The model under review builds one solid part; all positions refer to its coordinate system, in mm. A direction names the side the tool comes from. Give positions to 0.01 mm unless a question says otherwise; leave off trailing zeros. Order: outer loops, then holes, each group sorted by start corner. A loop starts at its lowest first (then second) coordinate and runs counter-clockwise, first axis right, second up. Notation, with made-up numbers: (85.5, -14.75) - (105.5, -14.75) arc R11 cw to (105.5, 2.25) - close; hole circle Ø11 at (66, -30.5). An arc over 180 degrees is marked (long way). Answer as CSV lines item,"result". Start each with the question number.
from build123d import *

# Parameters (mm, degrees)
BOSS_EXTRUDE1_DEPTH     = 8
SKETCH3_OUTSIDE_W       = 33.14
SKETCH3_OUTSIDE_H       = 32.15
SKETCH3_OUTSIDE_R       = 3.2
CUT_EXTRUDE1_DEPTH      = 10
CUT_EXTRUDE1_DRAFT      = -45
MIRROR2_COPY_1_SKETCH_W = 33.14
MIRROR2_COPY_1_SKETCH_H = 32.15
MIRROR2_COPY_1_SKETCH_R = 3.2
MIRROR2_COPY_1_DEPTH    = 10
MIRROR2_COPY_1_DRAFT    = -45


with BuildPart() as part:
    # Sketch1 → Boss-Extrude1 (new, symmetric)
    with BuildSketch(Plane(origin=(0, 0, 0), x_dir=(1, 0, 0), z_dir=(0, 1, 0))):
        Polygon((3.695041723, 0), (1.847520861, 3.2), (-1.847520861, 3.2), (-3.695041723, 0), (-1.847520861, -3.2), (1.847520861, -3.2), align=None)
    extrude(amount=BOSS_EXTRUDE1_DEPTH, both=True)


with BuildPart() as cut_extrude1_tool:
    # Sketch3 outside → Cut-Extrude1 (with draft: the straight prism first)
    with BuildSketch(Plane(origin=(0, 8, 0), x_dir=(1, 0, 0), z_dir=(0, 1, 0))):
        Rectangle(SKETCH3_OUTSIDE_W, SKETCH3_OUTSIDE_H)
        Circle(SKETCH3_OUTSIDE_R, mode=Mode.SUBTRACT)
    extrude(amount=-CUT_EXTRUDE1_DEPTH)
    # Cut-Extrude1: the draft: its side faces are tilted about the plane it starts from
    cut_extrude1_sides = [cut_extrude1_tool.faces().sort_by_distance(p)[0] for p in [
        (0, 3, 16.075),
        (16.57, 3, 0),
        (0, 3, -16.075),
        (-16.57, 3, 0),
        (-3.2, 3, 0),
    ]]
    draft(cut_extrude1_sides, Plane(origin=(0, 8, 0), x_dir=(1, 0, 0), z_dir=(0, 1, 0)), CUT_EXTRUDE1_DRAFT)


with BuildPart() as part_1:
    add(part.part)

    # Cut-Extrude1: cut by cut_extrude1_tool
    add(cut_extrude1_tool.part, mode=Mode.SUBTRACT)


with BuildPart() as mirror2_copy_1_tool:
    # Mirror2 copy 1 sketch → Mirror2 copy 1 (with draft: the straight prism first)
    with BuildSketch(Plane.XZ.offset(8)):
        Rectangle(MIRROR2_COPY_1_SKETCH_W, MIRROR2_COPY_1_SKETCH_H)
        Circle(MIRROR2_COPY_1_SKETCH_R, mode=Mode.SUBTRACT)
    extrude(amount=-MIRROR2_COPY_1_DEPTH)
    # Mirror2 copy 1: the draft: its side faces are tilted about the plane it starts from
    mirror2_copy_1_sides = [mirror2_copy_1_tool.faces().sort_by_distance(p)[0] for p in [
        (0, -3, 16.075),
        (16.57, -3, 0),
        (0, -3, -16.075),
        (-16.57, -3, 0),
        (-3.2, -3, 0),
    ]]
    draft(mirror2_copy_1_sides, Plane.XZ.offset(8), MIRROR2_COPY_1_DRAFT)


with BuildPart() as part_2:
    add(part_1.part)

    # Mirror2 copy 1: cut by mirror2_copy_1_tool
    add(mirror2_copy_1_tool.part, mode=Mode.SUBTRACT)

    # Sketch2 → M2.5 Tapped Hole1 (revolve, cut)
    with BuildSketch(Plane(origin=(0, 8, 0), x_dir=(0, 0, 1), z_dir=(1, 0, 0))):
        Polygon((0, 0), (0, 6.965882135), (1.025, 6.35), (1.025, 0), align=None)
    m2_5_tapped_hole1 = revolve(axis=Axis((0, 14.35, 0), (0, -1, 0)), mode=Mode.SUBTRACT)

    # Mirror1: M2.5 Tapped Hole1 across plane
    add(m2_5_tapped_hole1.mirror(Plane.ZX), mode=Mode.SUBTRACT)


solid = part_2.part
Item 1: Mouldability with a two-part tool opening along Z and no side actions: class faces 1 (the face through (1.65, -7.88, -2.88)), 2 (the face through (-2.784, 0.112, 1.578)), 3 (the face through (-0.05, 1.14, 0.17)), 4 (the face through (-0.05, -1.14, 0.17)) as released by +Z, released by -Z, zero draft, split by the parting line, or undercut.
Item 2: Machinability: for faces 5 (the face through (1.67, -7.88, 2.87)), 6 (the face through (-1.016, 4.869, -0.133)), which of the approach directions +Z, -Z, +X, -X, +Y, -Y give a long, thin tool a straight path to every point of the face, cutting with its end or side? Answer none if there is none.
Item 3: For line 1 along Z through (x, y) = (0, 4) (3 decimals); line 2 along X through (y, z) = (-5.5, 0.5); line 3 along X through (y, z) = (1.5, 0.25), list the stretches that pass through material, from the lowest coordinate up.
Item 4: Take a section at B-B on y = 0.25. Write out the cut boundary in (x, z), and give its area (3 significant figures).
Item 5: Take a section at A-A on y = -6.5. Write out the cut boundary in (x, z) (3 decimals), and give its area (3 significant figures).
Data:
1,face 1,"released by -Z"
1,face 2,"released by +Z"
1,face 3,"undercut"
1,face 4,"undercut"
2,face 5,"+Z, +X, -Y"
2,face 6,"+Y"
3,line 1,"z = -3.2 to -1.025, 1.025 to 3.2"
3,line 2,"x = -3.41 to -0.89, 0.89 to 3.41"
3,line 3,"x = -3.55 to -0.73, 0.73 to 3.55"
4,outline,"(-3.7, 0) - (-1.85, -3.2) - (1.85, -3.2) - (3.7, 0) - (1.85, 3.2) - (-1.85, 3.2) - close"
4,area,"35.5 mm^2"
5,outline,"(-3.695, 0) - (-1.848, -3.2) - (1.848, -3.2) - (3.695, 0) - (1.848, 3.2) - (-1.848, 3.2) - close; hole circle Ø2.05 at (0, 0)"
5,area,"32.2 mm^2"
